Input: part model. Units: mm. Frame: model coordinates. Coordinates: 2 decimals unless noted, no trailing zeros. Order: outer loops, then holes, each group sorted by start corner. A loop starts at its lowest first (then second) coordinate and runs counter-clockwise, first axis right, second up.
from build123d import *

# Parameters (mm, degrees)
F2_R = 10
F3_R = 2.5


with BuildPart() as f1:
    # F0 (on Front) → F1 (revolve)
    with BuildSketch(Plane.XZ):
        with BuildLine():
            Line((67.052818, 100), (63, 100))
            Line((63, 100), (47.347826, 4))
            Line((47.347826, 4), (0, 4))
            Line((0, 4), (0, 0))
            Line((0, 0), (50.74847, 0))
            Line((50.74847, 0), (61.995092, 68.979285))
            ThreePointArc((61.995092, 68.979285), (62.689931, 71.34783), (63.943775, 73.47402))
            ThreePointArc((63.943775, 73.47402), (64.430945, 74.597703), (64.325935, 75.817938))
            ThreePointArc((64.325935, 75.817938), (63.812397, 78.232288), (63.905895, 80.698877))
            Line((63.905895, 80.698877), (64.877049, 86.655283))
            ThreePointArc((64.877049, 86.655283), (66.341543, 91.562766), (69.004327, 95.937434))
            ThreePointArc((69.004327, 95.937434), (69.306305, 98.582494), (67.052818, 100))
        make_face()
    revolve(axis=Axis((0, 0, 51), (0, 0, 1)))

    # F2
    f2_edges = [f1.edges().sort_by_distance(p)[0] for p in [
        (-47.347826, 0, 4),
    ]]
    fillet(f2_edges, radius=F2_R)

    # F3
    f3_edges = [f1.edges().sort_by_distance(p)[0] for p in [
        (-63, 0, 100),
    ]]
    fillet(f3_edges, radius=F3_R)


solid = f1.part
Item 1: Pin query (flat end, axial travel): pin 1 Ø6 at (x, y) = (-30, -11.5) entering from +Z; pin 2 Ø1.5 at (y, z) = (-26.5, 16) entering from +X; pin 3 Ø12 at (y, z) = (44, 20.5) entering from -X; pin 4 Ø2 at (x, y) = (45.5, 55) entering from +Z. Return the tip coordinate at first contact, or that it passes through.
Response values:
pin 1: stops at z = 4
pin 2: stops at x = 46.76
pin 3: stops at x = -38.65
pin 4: passes through
Item 2: Cut plane A-A on x = 0. Return loops of the section in (y, z).
Response values:
outline: (-69, 95.94) arc R20 cw to (-64.88, 86.66) - (-63.91, 80.7) arc R10 cw to (-64.33, 75.82) arc R2.5 ccw to (-63.94, 73.47) arc R10 cw to (-62, 68.98) - (-50.75, 0) - (50.75, 0) - (62, 68.98) arc R10 cw to (63.94, 73.47) arc R2.5 ccw to (64.33, 75.82) arc R10 cw to (63.91, 80.7) - (64.88, 86.66) arc R20 cw to (69, 95.94) arc R2.5 ccw to (67.05, 100) - (65.13, 100) arc R2.5 ccw to (62.66, 97.9) - (48.72, 12.39) arc R10 cw to (38.85, 4) - (-38.85, 4) arc R10 cw to (-48.72, 12.39) - (-62.66, 97.9) arc R2.5 ccw to (-65.13, 100) - (-67.05, 100) arc R2.5 ccw to start
Item 3: Cut plane D-D on z = 42.5. Return loops of the section in (x, y) (3 decimals), then the cut area to 3 significant figures.
Response values:
outline: circle Ø115.356 at (0, 0); hole circle Ø107.25 at (0, 0)
area: 1,420 mm2
Item 4: Draft query along Z for faces 1 (the face through (61.013, 19.214, 81.071)), 2 (the face through (1, 1, 0)), 3 (the face through (-1, 1, 4)). Return one class per face: pulls with the +Z half, pulls with the -Z half, needs draft (parallel to the pull), parting line crosses it, or undercut.
Response values:
face 1: undercut
face 2: pulls with the -Z half
face 3: pulls with the +Z half
Item 5: Cut plane B-B on z = 67. Return loops of the section in (x, y), then the cut area to 3 significant figures.
Response values:
outline: circle Ø123.34 at (0, 0); hole circle Ø115.24 at (0, 0)
area: 1,520 mm2
Item 6: Ray query, probe 1 along Z at (x, y) = (-22, 23.5); probe 2 along X at (y, z) = (-26.5, 52.5); probe 3 along X at (y, z) = (43, 78). Return the intervals inside material, ascending.
Response values:
probe 1: z = 0 to 4
probe 2: x = -53.06 to -48.49, 48.49 to 53.06
probe 3: x = -47.18 to -41, 41 to 47.18
